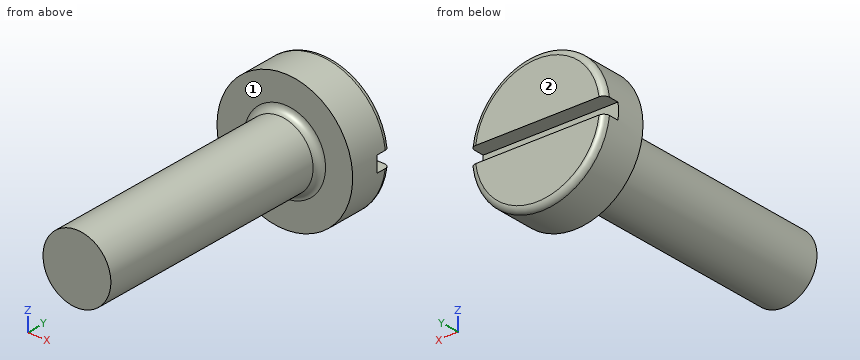
Autodesk Inventor part; units mm, degrees
ref_plane "YZ Plane" through (0, 0, 0) normal (1, 0, 0) x (0, 1, 0)
ref_plane "XZ Plane" through (0, 0, 0) normal (0, 1, 0) x (-1, 0, 0)
ref_plane "XY Plane" through (0, 0, 0) normal (0, 0, 1) x (1, 0, 0)
sketch "Sketch1" plane through (0, 0, 0) normal (0, 0, 1) x (1, 0, 0)
  line L0 (0, 0) -> (-1.5, 0)
  line L1 (-1.5, 0) -> (-1.5, 10)
  line L2 (-1.5, 10) -> (-1.5, 10)
  line L3 (-1.5, 10) -> (-1.5, 11)
  line L4 (-1.5, 11) -> (-3, 11)
  line L5 (-3, 11) -> (-3, 13)
  line L6 (-3, 13) -> (0, 13)
  line L7 (0, 13) -> (0, 0)
  dimension "d0" = 2
  dimension "d1" = 3
  dimension "d2" = 1.5
  dimension "d3" = 0
  dimension "d4" = 1
  dimension "d5" = 13
  dimension "d6" = 90
revolve "Revolution1" add sketch "Sketch1" angle 360 about axis through (0, 13, 0) along (0, -1, 0)
thread "Thread1"
sketch "Sketch2" plane through (0, 13, 0) normal (0, 1, 0) x (1, 0, 0)
  line L0 (5, 0.35) -> (-5, 0.35)
  line L1 (-5, 0.35) -> (-5, -0.35)
  line L2 (-5, -0.35) -> (5, -0.35)
  line L3 (5, -0.35) -> (5, 0.35)
  line L4 (5, 0.35) -> (-5, -0.35) construction
  line L5 (-5, 0.35) -> (5, -0.35) construction
  point P0 (0, 0)
  dimension "d10" = 10
  dimension "d11" = 0.7
fillet "Fillet1" radius 0.25 1 edges at (3, 13, 0)
extrude "Extrusion2" cut sketch "Sketch2" against normal blind 0.7
fillet "Fillet2" radius 0.3 1 edges at (1.5, 11, 0)
properties part number "TorsionOscillator-Screw-M3-Brass-CheeseHead-10mm-fine" material "Brass, Soft Yellow"
Input: part model. Units: mm. Frame: model coordinates. Face numbers are marked on the shaded views. A direction names the side the tool comes from. Coordinates: 2 decimals unless noted, no trailing zeros. Write each loop counter-clockwise with the first axis right and the second up, starting at its lowest first coordinate (ties: lowest second). Pieces come first, ordered by that corner, then holes. Notation, with made-up numbers: (88.25, 26.25) -> (102.25, 26.25) arc R20 ccw to (102.25, 39.25) -> close; hole circle Ø11 at (-20, 61.25). An arc over 180 degrees is marked (long way). Answer as a JSON object with one key per item and string values.
1. Access query for the marked faces 1 and 2. Directions: +Z, -Z, +X, -X, +Y, -Y. A direction counts if a zero-diameter tool reaches every point of the face in a straight line with its end or side. Return the directions, or none.
Result set:
{"face 1": "-Y", "face 2": "+Z, -Z, +X, -X, +Y"}
2. Section D-D on y = 12. Return the cut outline in (x, z).
Result set:
{"outline": "circle Ø6 at (0, 0)"}
3. Section C-C on y = 8. Return the cut outline in (x, z), then the cut area to 3 significant figures.
Result set:
{"outline": "circle Ø3 at (0, 0)", "area": "7.07 mm2"}
4. Section B-B on x = 0. Return the cut outline in (y, z).
Result set:
{"outline": "(0, -1.5) -> (10.7, -1.5) arc R0.3 cw to (11, -1.8) -> (11, -3) -> (12.75, -3) arc R0.25 ccw to (13, -2.75) -> (13, -0.35) -> (12.3, -0.35) -> (12.3, 0.35) -> (13, 0.35) -> (13, 2.75) arc R0.25 ccw to (12.75, 3) -> (11, 3) -> (11, 1.8) arc R0.3 cw to (10.7, 1.5) -> (0, 1.5) -> close"}
5. Section A-A on z = 0. Return the cut outline in (x, y), then the cut area to 3 significant figures.
Result set:
{"outline": "(-3, 11) -> (-1.8, 11) arc R0.3 cw to (-1.5, 10.7) -> (-1.5, 0) -> (1.5, 0) -> (1.5, 10.7) arc R0.3 cw to (1.8, 11) -> (3, 11) -> (3, 12.3) -> (-3, 12.3) -> close", "area": "40.8 mm2"}
6. Material intervals for line 1 (Y direction, x = 0.8, z = 1.75); line 2 (Y direction, x = -2.7, z = 0); line 3 (Z direction, x = 2.15, y = 12.5), sorted ascending. Write a range as from..to.
Result set:
{"line 1": "y = 11..13", "line 2": "y = 11..12.3", "line 3": "z = -2.09..-0.35, 0.35..2.09"}
7. First-contact query: P1, Ø1.5, axis at x = -1, y = 6, coming from the -Z side; P2, Ø0.6, axis at x = -1, y = 12.5, coming from the -Z side; P3, Ø0.6, axis at x = -0.5, y = 12.5, coming from the +Z side. Flat tips, straight axial feed; report the tip coordinate or a pass-through.
Result set:
{"P1": "stops at z = -1.48", "P2": "stops at z = -2.92", "P3": "stops at z = 2.99"}
